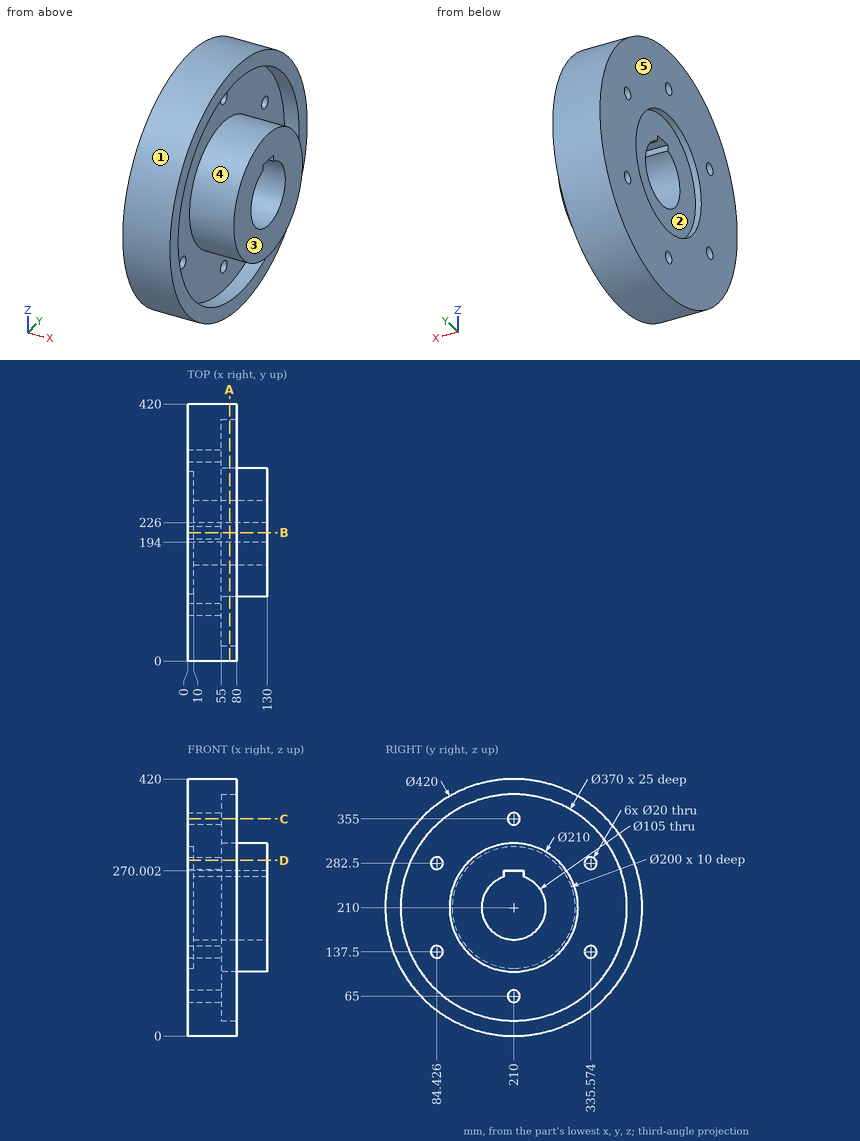
Source: three-view drawing plus pictorial views. Frame: mm from the lowest corner of the part. A direction names the side the tool comes from. Give positions to 0.01 mm unless a question says otherwise; leave off trailing zeros. Write each loop counter-clockwise with the first axis right and the second up, starting at its lowest first coordinate (ties: lowest second). Pieces come first, ordered by that corner, then holes. Notation, with made-up numbers: (77, -31.5) - (83, -31.5) arc R29 cw to (83, -11.5) - close; hole circle Ø11 at (4.5, 41). An arc over 180 degrees is marked (long way). Write item = value, one per line. Start each with the question number.
1. Ray query, L1, parallel to Z at x = 61, y = 210; L2, parallel to Y at x = 7, z = 210; L3, parallel to Y at x = 62, z = 210. Return the intervals inside material, ascending.
2. Access query for the marked faces 4 and 5. Directions: +Z, -Z, +X, -X, +Y, -Y. A direction counts if a zero-diameter tool reaches every point of the face in a straight line with its end or side. Return the directions, or none.
3. First-contact query: pin 1 Ø4 at (y, z) = (136.5, 225) entering from -X; pin 2 Ø8 at (x, z) = (88, 263) entering from +Y (1 decimal); pin 3 Ø3 at (y, z) = (102, 244.5) entering from +X; pin 4 Ø18 at (y, z) = (210, 355) entering from -X. Flat tips, straight axial feed; report the tip coordinate or a pass-through.
4. Section query D-D, the plane z = 287. Output: boundary loops of the cut face in (x, y) (1 decimal).
5. Section query A-A, the plane x = 68.5. Output: boundary loops of the cut face in (y, z).
6. Section query C-C, the plane z = 355. Output: boundary loops of the cut face in (x, y) (1 decimal).
7. Mould query, pull axis Y, two halves, no side actions, for the marked faces 1, 2 and 3. Classes: released by +Y, released by -Y, zero draft, split by the parting line, or undercut.
8. Section query B-B, the plane y = 210. Output: boundary loops of the cut face in (x, z).
Check sheet entries:
q1.L1 = 0 to 25, 105 to 157.5, 270 to 315, 395 to 420
q1.L2 = 0 to 110, 310 to 420
q1.L3 = 0 to 25, 105 to 157.5, 262.5 to 315, 395 to 420
q2.face_4 = +X
q2.face_5 = +Z, -Z, -X, +Y, -Y
q3.pin_1 = 10
q3.pin_2 = 302.9
q3.pin_3 = 55
q3.pin_4 = through
q4.outline = (0, 14.6) - (80, 14.6) - (80, 41.8) - (55, 41.8) - (55, 75.5) - (0, 75.5) - close; (0, 93.4) - (55, 93.4) - (55, 138.6) - (130, 138.6) - (130, 281.4) - (55, 281.4) - (55, 326.6) - (0, 326.6) - (0, 273.8) - (10, 273.8) - (10, 146.2) - (0, 146.2) - close; (0, 344.5) - (55, 344.5) - (55, 378.2) - (80, 378.2) - (80, 405.4) - (0, 405.4) - close
q5.outline = circle Ø420 at (210, 210); circle Ø210 at (210, 210); hole circle Ø370 at (210, 210); hole (194, 260) arc R52.5 ccw (long way) to (226, 260) - (226, 270) - (194, 270) - close
q6.outline = (0, 58.1) - (80, 58.1) - (80, 95.1) - (55, 95.1) - (55, 200) - (0, 200) - close; (0, 220) - (55, 220) - (55, 324.9) - (80, 324.9) - (80, 361.9) - (0, 361.9) - close
q7.face_1 = split by the parting line
q7.face_2 = undercut
q7.face_3 = zero draft
q8.outline = (0, 0) - (80, 0) - (80, 25) - (55, 25) - (55, 55) - (0, 55) - close; (0, 75) - (55, 75) - (55, 105) - (130, 105) - (130, 157.5) - (10, 157.5) - (10, 110) - (0, 110) - close; (0, 310) - (10, 310) - (10, 270) - (130, 270) - (130, 315) - (55, 315) - (55, 345) - (0, 345) - close; (0, 365) - (55, 365) - (55, 395) - (80, 395) - (80, 420) - (0, 420) - close
